For this review, take the finished solid that the model builds, in its own axes (mm). Face numbers are marked on the shaded views. Round coordinates to 2 decimals unless told otherwise and drop trailing zeros. Order: outer loops, then holes, each group sorted by start corner. A loop starts at its lowest first (then second) coordinate and runs counter-clockwise, first axis right, second up. Notation, with made-up numbers: M -37,-5.5 L -3,-5.5 A22 cw -3,18.5 Z; hole C 73.5,82 d3. An arc over 180 degrees is marked long. Answer as a JSON object with one key per item and string values.
from build123d import *

# Parameters (mm, degrees)
F1_DEPTH = 10.9
F2_R     = 5
F3_R     = 5
F4_DEPTH = 25


with BuildPart() as f1:
    # F0 (on Top) → F1 (new body)
    with BuildSketch(Plane.XY):
        Polygon((-2.8653, -40.312819), (36.344576, 17.674987), (-33.479275, 22.637833), align=None)
    extrude(amount=F1_DEPTH)

    # F2
    f2_edges = [f1.edges().sort_by_distance(p)[0] for p in [
        (36.344576, 17.674987, 5.45),
        (-2.8653, -40.312819, 5.45),
        (-33.479275, 22.637833, 5.45),
    ]]
    fillet(f2_edges, radius=F2_R)

    # F3 (on face) → F4 (cut)
    with BuildSketch(Plane.XY.offset(10.9)):
        with Locations((-1.447344, -20.363147)):
            Circle(F3_R)
        with Locations((18.358675, 8.928137)):
            Circle(F3_R)
        with Locations((-16.911331, 11.435011)):
            Circle(F3_R)
    extrude(amount=-F4_DEPTH, mode=Mode.SUBTRACT)


solid = f1.part
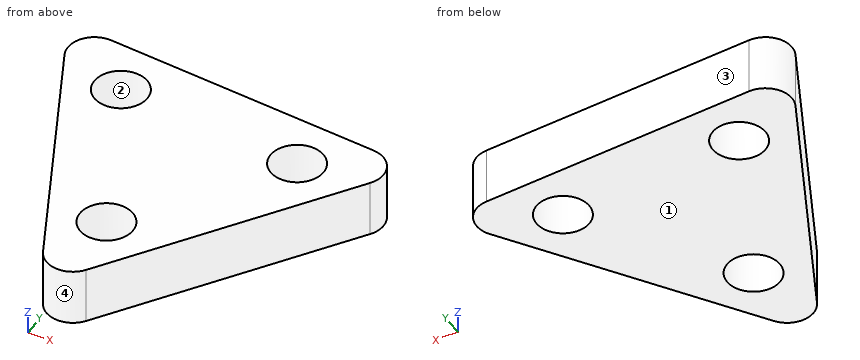
1) Mouldability with a two-part tool opening along X and no side actions: class the marked faces 1, 2, 3 and 4 as +X half, -X half, draft (parallel to the pull), parting line (faces both ways), or undercut.
Geometry check:
{"face 1": "draft", "face 2": "undercut", "face 3": "+X half", "face 4": "parting line"}
2) For L1, parallel to X at y = 13.5, z = 2 (3 decimals); L2, parallel to Y at x = -0.5, z = 10.25; L3, parallel to Y at x = -4, z = 3, list the stretches that pass through material, from the lowest coordinate up.
Geometry check:
{"L1": "x = -29.035 to -21.465, -12.358 to 16.334, 20.383 to 32.348", "L2": "y = -35.06 to -25.27, -15.45 to 20.29", "L3": "y = -34.99 to -24.66, -16.06 to 20.54"}
3) Add section A-A on x = -16.5. State the section outline as (y, z) points, and give its area (3 significant figures).
Geometry check:
{"outline": "M -12.28,0 L 6.45,0 L 6.45,10.9 L -12.28,10.9 Z; M 16.42,0 L 21.43,0 L 21.43,10.9 L 16.42,10.9 Z", "area": "259 mm²"}
4) Add section C-C on z = 6. State the section outline as (x, y) points, and give its area (3 significant figures).
Geometry check:
{"outline": "M -29.69,14.85 L -6.65,-32.52 A5 ccw 1.99,-33.14 L 31.49,10.5 A5 ccw 27.71,18.29 L -24.84,22.02 A5 ccw Z; hole C -16.91,11.44 d10; hole C -1.45,-20.36 d10; hole C 18.36,8.93 d10", "area": "1,830 mm²"}
5) Insertion check: P1, Ø6, axis at x = 10, z = 3, coming from the -Y side; P2, Ø2, axis at x = 23.5, z = 9, coming from the +Y side; P3, Ø9, axis at x = -1.45, y = -20.36, coming from the +Z side; P4, Ø2, axis at x = -9, z = 2.5, coming from the +Y side. Each pin has a flat end and moves straight along its axis. Give the tip position at first contact, or say it passes through.
Geometry check:
{"P1": "stops at y = -25.72", "P2": "stops at y = 18.66", "P3": "passes through", "P4": "stops at y = 20.97"}
6) Add section D-D on y = -29.5. State the section outline as (x, z) points, and give its area (3 significant figures).
Geometry check:
{"outline": "M -8.12,0 L 4.45,0 L 4.45,10.9 L -8.12,10.9 Z", "area": "137 mm²"}
7) Add section B-B on y = -17. State the section outline as (x, z) points.
Geometry check:
{"outline": "M -14.2,0 L -5.15,0 L -5.15,10.9 L -14.2,10.9 Z; M 2.25,0 L 12.9,0 L 12.9,10.9 L 2.25,10.9 Z"}
